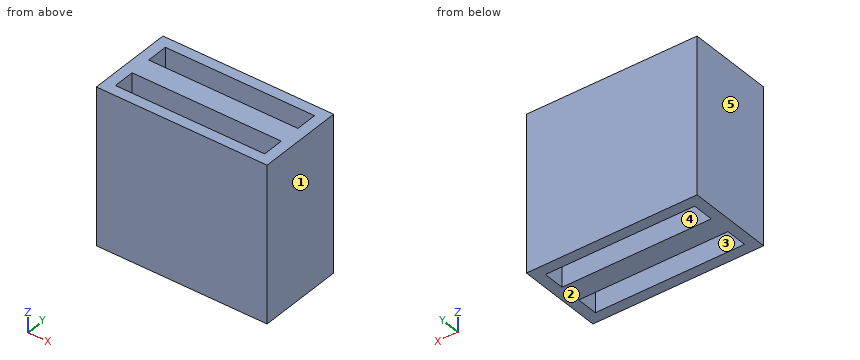
```python
from build123d import *

# Parameters (mm, degrees)
F0_W     = 100.84179
F0_H     = 92.084482
F1_DEPTH = 50.8
F2_W     = 88.14179
F2_H     = 12.7
F3_DEPTH = 101.6


with BuildPart() as f1:
    # F0 (on Front) → F1 (new body)
    with BuildSketch(Plane.XZ):
        Rectangle(F0_W, F0_H)
    extrude(amount=F1_DEPTH)

    # F2 (on face) → F3 (cut)
    with BuildSketch(Plane.XY.offset(46.042241)):
        with Locations((0, -12.7)):
            Rectangle(F2_W, F2_H)
        with Locations((0, -38.1)):
            Rectangle(F2_W, F2_H)
    extrude(amount=-F3_DEPTH, mode=Mode.SUBTRACT)


solid = f1.part
```
Work out the finished part from the listing and answer in its coordinate system (mm). Face numbers are marked on the shaded views. A direction names the side the tool comes from. Coordinates: 2 decimals unless noted, no trailing zeros. Write each loop counter-clockwise with the first axis right and the second up, starting at its lowest first coordinate (ties: lowest second). Pieces come first, ordered by that corner, then holes. Notation, with made-up numbers: (-19.5, 15) - (-4.5, 15) arc R19 ccw to (-4.5, 51) - close; hole circle Ø11 at (-3, 40.5). An arc over 180 degrees is marked (long way). Answer as a JSON object with one key per item and string values.
Q1. Consider L1, parallel to Y at x = -43.5, z = 29; L2, parallel to X at y = -36, z = -27. Determine where each line is inside the solid, lowest interval first. Write a range as from..to.
Results list:
{"L1": "y = -50.8..-44.45, -31.75..-19.05, -6.35..0", "L2": "x = -50.42..-44.07, 44.07..50.42"}
Q2. Find section C-C (x = 31.5). Write down the section's boundary in (y, z).
Results list:
{"outline": "(-50.8, -46.04) - (-44.45, -46.04) - (-44.45, 46.04) - (-50.8, 46.04) - close; (-31.75, -46.04) - (-19.05, -46.04) - (-19.05, 46.04) - (-31.75, 46.04) - close; (-6.35, -46.04) - (0, -46.04) - (0, 46.04) - (-6.35, 46.04) - close"}
Q3. Find section B-B (z = 33). Write down the section's boundary in (x, y), plus the area to 3 significant figures.
Results list:
{"outline": "(-50.42, -50.8) - (50.42, -50.8) - (50.42, 0) - (-50.42, 0) - close; hole (-44.07, -44.45) - (44.07, -44.45) - (44.07, -31.75) - (-44.07, -31.75) - close; hole (-44.07, -19.05) - (44.07, -19.05) - (44.07, -6.35) - (-44.07, -6.35) - close", "area": "2,880 mm^2"}
Q4. Which of the six approach directions +Z, -Z, +X, -X, +Y, -Y give full straight-line access (tool end or side, diameter ignored) to the marked faces 4 and 5?
Results list:
{"face 4": "+Z, -Z", "face 5": "+Z, -Z, -X, +Y, -Y"}
Q5. Find section A-A (y = -34). Write down the section's boundary in (x, z), plus the area to 3 significant figures.
Results list:
{"outline": "(-50.42, -46.04) - (-44.07, -46.04) - (-44.07, 46.04) - (-50.42, 46.04) - close; (44.07, -46.04) - (50.42, -46.04) - (50.42, 46.04) - (44.07, 46.04) - close", "area": "1,170 mm^2"}
Q6. For a pull along X with two mould halves and no side action, classify the marked faces 1, 2 and 3 as pulls with the +X half, pulls with the -X half, needs draft (parallel to the pull), parting line crosses it, or undercut.
Results list:
{"face 1": "pulls with the +X half", "face 2": "needs draft", "face 3": "undercut"}
